CAD build for the part. Positions are in the model's coordinates, mm. Face numbers are marked on the shaded views. A direction names the side the tool comes from. Give positions to 0.01 mm unless a question says otherwise; leave off trailing zeros. Loops run counter-clockwise (first coordinate to the right, second up) from the corner with the lowest first, then second, coordinate; pieces in that order, holes last. Notation, with made-up numbers: (1.25, 56) -> (6.25, 56) arc R18 ccw to (6.25, 62) -> close; hole circle Ø2 at (34, -19.75). An arc over 180 degrees is marked (long way). Use one line per item in the form item = value.
```python
from build123d import *

# Parameters (mm, degrees)
SKETCH2_W               = 104
SKETCH2_H               = 115
BOSS_EXTRUDE1_DEPTH     = 104
CUT_EXTRUDE1_DEPTH      = 187.70029459
CUT_EXTRUDE2_DEPTH      = 187.70029459
SKETCH5_R               = 25
CUT_EXTRUDE3_DEPTH      = 187.70029459
SKETCH7_R               = 40
CUT_EXTRUDE4_DEPTH      = 10
FILLET1_R               = 15
SKETCH8_W               = 52
SKETCH8_H               = 52
CUT_EXTRUDE5_DEPTH      = 187.70029459
CUT_EXTRUDE6_DEPTH      = 187.70029459
CUT_EXTRUDE6_DEPTH_BACK = 10


with BuildPart() as part:
    # Sketch2 → Boss-Extrude1 (new body)
    with BuildSketch(Plane.XY):
        with Locations((52, 57.5)):
            Rectangle(SKETCH2_W, SKETCH2_H)
    extrude(amount=BOSS_EXTRUDE1_DEPTH)

    # Sketch3 → Cut-Extrude1 (cut, through all)
    with BuildSketch(Plane.XY.offset(104)):
        Polygon((0, 115), (24.407301932, 57.5), (0, 0), align=None)
        Polygon((104, 115), (79.592698068, 57.5), (104, 0), align=None)
    extrude(amount=-CUT_EXTRUDE1_DEPTH, mode=Mode.SUBTRACT)

    # Sketch4 → Cut-Extrude2 (cut, through all)
    with BuildSketch(Plane(origin=(0, 0, 0), x_dir=(0, 0, -1), z_dir=(1, 0, 0))):
        Polygon((-104, 115), (-79.592698068, 57.5), (-104, 0), align=None)
        Polygon((0, 115), (-24.407301932, 57.5), (0, 0), align=None)
    extrude(amount=CUT_EXTRUDE2_DEPTH, mode=Mode.SUBTRACT)

    # Sketch5 → Cut-Extrude3 (cut, through all)
    with BuildSketch(Plane(origin=(0, 115, 0), x_dir=(1, 0, 0), z_dir=(0, 1, 0))):
        with Locations(Location((52, -52, 0), (0, 0, 270))):
            Circle(SKETCH5_R)
    extrude(amount=-CUT_EXTRUDE3_DEPTH, mode=Mode.SUBTRACT)

    # Sketch7 → Cut-Extrude4 (cut)
    with BuildSketch(Plane(origin=(0, 115, 0), x_dir=(1, 0, 0), z_dir=(0, 1, 0))):
        with Locations(Location((52, -52, 0), (0, 0, 270))):
            Circle(SKETCH7_R)
    extrude(amount=-CUT_EXTRUDE4_DEPTH, mode=Mode.SUBTRACT)

    # Fillet1
    fillet1_edges = [part.edges().sort_by_distance(p)[0] for p in [
        (24.407301932, 57.5, 52),
        (79.592698068, 57.5, 52),
        (52, 57.5, 79.592698068),
        (52, 57.5, 24.407301932),
    ]]
    fillet(fillet1_edges, radius=FILLET1_R)

    # Sketch8 → Cut-Extrude5 (cut, through all)
    with BuildSketch(Plane(origin=(0, 115, 0), x_dir=(1, 0, 0), z_dir=(0, 1, 0))):
        with Locations((78, -78)):
            Rectangle(SKETCH8_W, SKETCH8_H)
    extrude(amount=-CUT_EXTRUDE5_DEPTH, mode=Mode.SUBTRACT)

    # Sketch9 → Cut-Extrude6 (cut, two sides: drawn at the far end of the back side and taken through both)
    with BuildSketch(Plane.XZ.offset(-CUT_EXTRUDE6_DEPTH_BACK)):
        with BuildLine():
            Line((52, 77), (52, 92))
            ThreePointArc((52, 92), (23.715728753, 23.715728753), (92, 52))
            Line((92, 52), (77, 52))
            ThreePointArc((77, 52), (34.32233047, 34.32233047), (52, 77))
        make_face()
    extrude(amount=CUT_EXTRUDE6_DEPTH + CUT_EXTRUDE6_DEPTH_BACK, mode=Mode.SUBTRACT)


solid = part.part
```
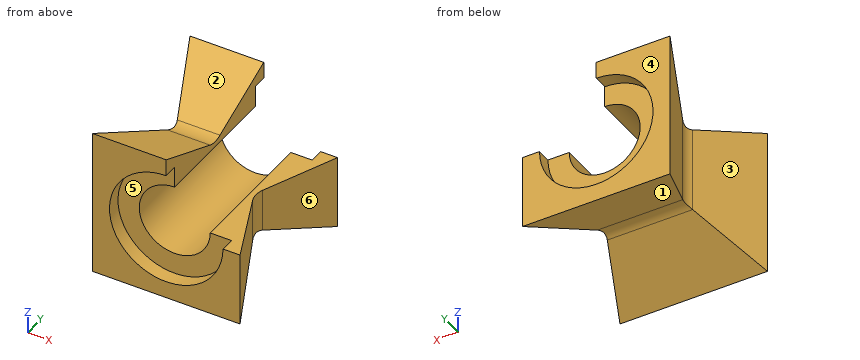
1. Tool access for the marked faces 1, 2 and 3: list every direction of +Z, -Z, +X, -X, +Y, -Y with a clear straight run to the whole face (end or side of a thin tool).
Result sheet:
face_1 = -Z, +X, -X
face_2 = +Z, +X, -X
face_3 = +Z, -Z, -X
2. Drill centre lines: line 1 (Y direction, x = 4.5, z = 60); line 2 (Y direction, x = 97, z = 8); line 3 (X direction, y = 34, z = 39.5). Where is each one in solid material? Low to high.
Result sheet:
line_1 = 0 to 10.6, 104.4 to 115
line_2 = 0 to 16.49, 98.51 to 115
line_3 = 14.43 to 30.35, 73.65 to 89.57
3. Cut at B-B, the plane x = 13.5. Write the cut outline in (y, z).
Result sheet:
outline = (0, 0) -> (31.8, 13.5) -> (31.8, 90.5) -> (0, 104) -> (0, 62.85) -> (10, 62.85) -> (10, 41.15) -> (0, 41.15) -> close; (83.2, 13.5) -> (115, 0) -> (115, 41.15) -> (105, 41.15) -> (105, 62.85) -> (115, 62.85) -> (115, 104) -> (83.2, 90.5) -> close
4. Mould opens along X. For the marked faces 4, 5 and 6 say: pulls with the +X half, pulls with the -X half, needs draft (parallel to the pull), parting line crosses it, or undercut.
Result sheet:
face_4 = needs draft
face_5 = undercut
face_6 = pulls with the +X half
5. Cut at A-A, the plane z = 95. Write the cut outline in (x, y).
Result sheet:
outline = (0, 0) -> (52, 0) -> (52, 21.2) -> (9, 21.2) -> close; (0, 115) -> (9, 93.8) -> (52, 93.8) -> (52, 115) -> close
6. Cut at D-D, the plane z = 56. Write the cut outline in (x, y).
Result sheet:
outline = (0, 0) -> (12.2, 0) -> (12.2, 10) -> (27.32, 10) -> (27.32, 105) -> (12.2, 105) -> (12.2, 115) -> (0, 115) -> (21.92, 63.36) arc R15 cw to (21.92, 51.64) -> close
7. Drop flat-ended pins along their axis: P1, Ø6, axis at x = 85, y = 24, coming from the -Z side; P2, Ø1.5, axis at x = 56.5, y = 37.5, coming from the -Z side; P3, Ø12, axis at x = 45, z = 74, coming from the -Y side; P4, Ø21.5, axis at x = 92.5, y = 59, coming from the +Z side. Give the stop position or say it passes through.
Result sheet:
P1 = 8.91
P2 = 15.6
P3 = 10
P4 = through
8. Cut at C-C, the plane y = 58. Write the cut outline in (x, z).
Result sheet:
outline = (23.1, 23.1) -> (80.9, 23.1) -> (80.9, 52) -> (77, 52) arc R25 cw (long way) to (52, 77) -> (52, 80.9) -> (23.1, 80.9) -> close
